Autodesk Inventor part; units mm, degrees
ref_plane "YZ Plane" through (0, 0, 0) normal (1, 0, 0) x (0, 1, 0)
ref_plane "XZ Plane" through (0, 0, 0) normal (0, 1, 0) x (-1, 0, 0)
ref_plane "XY Plane" through (0, 0, 0) normal (0, 0, 1) x (1, 0, 0)
sketch "スケッチ1" plane through (0, 0, 0) normal (1, 0, 0) x (0, 1, 0)
  line L0 (35, -40) -> (-5, -40)
  line L1 (-5, -40) -> (-5, -100)
  line L2 (-5, -100) -> (35, -100)
  line L3 (35, -100) -> (35, -40)
  circle A0 centre (15, 0) radius 17.5
  line L4 (35, -40) -> (32.4668, 1.0772)
  line L5 (-5, -40) -> (-2.4668, 1.0772)
  dimension "d1" = 40
  dimension "d2" = 60
  dimension "d54" = 35
  dimension "d55" = 20
extrude "押し出し1" add sketch "スケッチ1" along normal blind 3
sketch "スケッチ4" plane through (3, 0, 0) normal (1, 0, 0) x (0, 0, -1)
  line L0 (54, 30) -> (95, 30)
  line L1 (95, 30) -> (95, 0)
  line L2 (95, 0) -> (54, 0)
  line L3 (54, 0) -> (54, 30)
  line L4 (100, 35) -> (40, 35)
  line L5 (100, -5) -> (100, 35)
  point P0 (0, 0)
  dimension "d29" = 41
  dimension "d30" = 30
  dimension "d31" = 5
  dimension "d32" = 5
hole "穴2" at (3, 30, -54) at (3, 0, -54) at (3, 0, -95) at (3, 30, -95) direction (-1, 0, 0) diameter 3.2 end through all
sketch "スケッチ6" plane through (3, 0, 0) normal (1, 0, 0) x (0, 0, -1)
  arc A0 (-1.0772, 32.4668) -> (-1.0772, -2.4668) centre (0, 15) ccw
  circle A1 centre (0, 15) radius 13.5
  point P0 (0, 0)
  point P1 (0, 1.5)
  point P2 (11.6913, 8.25)
  point P3 (11.6913, 21.75)
  point P4 (0, 28.5)
  point P5 (-11.6913, 21.75)
  point P6 (-11.6913, 8.25)
  dimension "d56" = 27
  dimension "d59" = 360
hole "穴4" at (3, 1.5, 0) at (3, 8.25, -11.6913) at (3, 21.75, -11.6913) at (3, 28.5, 0) at (3, 21.75, 11.6913) at (3, 8.25, 11.6913) direction (-1, 0, 0) diameter 3.2 end through all
properties part number "link6_plate1" material "アルミニウム 6061"
Source: CAD feature listing. Evaluate the final solid. Frame: model axes, mm. Give positions to 0.01 mm unless a question says otherwise; leave off trailing zeros. Write each loop counter-clockwise with the first axis right and the second up, starting at its lowest first coordinate (ties: lowest second). Pieces come first, ordered by that corner, then holes. Notation, with made-up numbers: (71, 74.25) - (108, 74.25) arc R25 ccw to (108, 88.25) - close; hole circle Ø3 at (-4.5, 53). An arc over 180 degrees is marked (long way). Write item = value, one per line. Start each with the question number.
Q1. Draft query along Y for faces 1 (the cylindrical face through (1.479, 26.914, 0.208)), 2 (the flat face through (1, 15, -100)), 3 (the flat face through (1.48, 33.75, -19.75)). Return one class per face: +Y half, -Y half, draft (parallel to the pull), parting line (faces both ways), or undercut.
Q2. Cut plane C-C, the plane z = 0. Return loops of the section in (x, y), then the cut area to 3 significant figures.
Q3. Pin query (flat end, axial travel): pin 1 Ø3 at (y, z) = (30, -95) entering from +X; pin 2 Ø1 at (x, y) = (1, 10) entering from +Z. Return the tip coordinate at first contact, or that it passes through.
Q4. Cut plane B-B, the plane x = 1.05. Give the number of separate pieces and of enclosed holes in the cut face, then the cut area to 3 significant figures.
Q5. Cut plane A-A, the plane z = -95. Return loops of the section in (x, y), then the cut area to 3 significant figures.
Q6. Material intervals for probe 1 along Y at (x, z) = (1.15, 0); probe 2 along Z at (x, y) = (1.8, 8.25); probe 3 along Z at (x, y) = (1.15, 15), sorted ascending.
Computed values:
q1.face_1 = undercut
q1.face_2 = draft
q1.face_3 = +Y half
q2.outline = (0, -2.53) - (3, -2.53) - (3, -0.1) - (0, -0.1) - close; (0, 3.1) - (3, 3.1) - (3, 26.9) - (0, 26.9) - close; (0, 30.1) - (3, 30.1) - (3, 32.53) - (0, 32.53) - close
q2.area = 86.0 mm²
q3.pin_1 = through
q3.pin_2 = 16.91
q4.separate_pieces = 1
q4.enclosed_holes = 10
q4.area = 4,300 mm²
q5.outline = (0, -5) - (3, -5) - (3, -1.6) - (0, -1.6) - close; (0, 1.6) - (3, 1.6) - (3, 28.4) - (0, 28.4) - close; (0, 31.6) - (3, 31.6) - (3, 35) - (0, 35) - close
q5.area = 101 mm²
q6.probe_1 = -2.53 to -0.1, 3.1 to 26.9, 30.1 to 32.53
q6.probe_2 = -100 to -13.29, -10.09 to 10.09, 13.29 to 16.15
q6.probe_3 = -100 to 17.5
